Autodesk Inventor part; units mm, degrees
ref_plane "Work Plane1" through (0, 90, 0) normal (1, 0, 0) x (0, 1, 0)
ref_plane "YZ Plane" through (0, 0, 0) normal (1, 0, 0) x (0, 1, 0)
ref_plane "XZ Plane" through (0, 0, 0) normal (0, 1, 0) x (-1, 0, 0)
sketch "Sketch1" plane through (0, 0, 0) normal (1, 0, 0) x (0, 1, 0)
  line L0 (0, 0) -> (90, 0)
  line L1 (90, 0) -> (90, -90)
  line L2 (90, -90) -> (0, -90)
  line L3 (0, -90) -> (0, 0)
  dimension "d0" = 90
  dimension "d1" = 90
ref_plane "Work Plane1" through (0, 90, 0) normal (1, 0, 0) x (0, 1, 0)
sketch "Sketch2" plane through (0, 90, 0) normal (1, 0, 0) x (0, 1, 0)
  line L0 (20, -20) -> (-65, -20)
  line L1 (-65, -20) -> (-65, 0)
  line L2 (-65, 0) -> (-90, 0)
  line L3 (-90, 0) -> (-90, -90)
  line L4 (-90, -90) -> (-65, -90)
  line L5 (-65, -90) -> (-65, -70)
  line L6 (-65, -70) -> (20, -70)
  line L7 (20, -70) -> (20, -20)
  line L8 (0, -90) -> (0, 0)
  line L9 (0, 0) -> (0, -90)
  line L10 (-90, 0) -> (-90, -90)
  line L11 (0, -90) -> (-90, -90)
  line L12 (-90, -90) -> (-90, 0)
  line L13 (-90, 0) -> (0, 0)
  line L14 (0, -45) -> (-90, -45) construction
  circle A0 centre (0, -45) radius 10
  point P0 (20, -45)
  point P1 (-90, -45)
  point P2 (0, -70)
  point P3 (-65, 0)
  point P4 (0, -20)
  point P5 (0, -35)
  point P6 (0, -55)
  dimension "d4" = 90
  dimension "d7" = 50
  dimension "d10" = 20
  dimension "d11" = 90
  dimension "d13" = 25
  dimension "d14" = 25
  dimension "d27" = 110
ref_plane "Work Plane2" through (45, 110, -45) normal (0, 0, 1) x (1, 0, 0)
sketch "Sketch4" plane through (45, 110, -45) normal (0, 0, 1) x (1, 0, 0)
  line L0 (-90, 0) -> (0, 0)
  line L1 (-90, 0) -> (0, 0)
  line L2 (0, 0) -> (0, -110)
  line L3 (0, -110) -> (-90, -110)
  line L4 (-90, -110) -> (-90, 0)
  line L5 (-90, 0) -> (-75, 0)
  line L6 (-75, 0) -> (-15, 0)
  line L7 (-15, 0) -> (0, 0)
  line L8 (0, -110) -> (0, 0)
  line L9 (0, -110) -> (0, -85)
  line L10 (0, -85) -> (-90, -85)
  line L11 (-75, 0) -> (-75, -85)
  line L12 (-15, 0) -> (-15, -85)
  point P0 (-45, -110)
  dimension "d22" = 15
  dimension "d23" = 60
  dimension "d24" = 25
  dimension "d28" = 110
extrude "Extrusion6" add sketch "Sketch2" along normal mid plane 90 contours L7 L6 L8 A0 L0 | L8 A0 L6 L5 L4 L3 L2 L1 L0
extrude "Extrusion7" cut sketch "Sketch4" along normal mid plane 90 contours L0 L12 L10 L11
properties part number "CT_01"
Read the model definition and answer for the solid it produces. Units are mm, in the model's axes. A direction names the side the tool comes from. Round coordinates to 2 decimals unless told otherwise and drop trailing zeros. Loops run counter-clockwise (first coordinate to the right, second up) from the corner with the lowest first, then second, coordinate; pieces in that order, holes last.
Q1. Consider probe 1 along X at (y, z) = (67, -62); probe 2 along Z at (x, y) = (36, 90); probe 3 along Y at (x, z) = (33.75, -45). Determine where each line is inside the solid, lowest interval first.
Q2. Section A-A on y = 62.5 is taken. Write down the section's boundary in (x, z).
Q3. Section D-D on z = -25 is taken. Write down the section's boundary in (x, y), and give its area (3 significant figures).
Q4. Determine the mould class of faces 1 (the face through (-45, 42, -44)), 2 (the face through (-1, 25, -46)), 3 (the face through (37, 68, -20)) for opening direction X: released by +X, released by -X, zero draft, split by the parting line, or undercut.
Q5. Each of these flat-tipped pins is pushed along its axis until it touches: pin 1 (12 mm diameter, centred on x = -40.5, y = 54, fed in from -Z); pin 2 (16.5 mm diameter, centred on x = 38.5, y = 83.5, fed in from +Z); pin 3 (18 mm diameter, centred on y = 90, z = -45, fed in from +X) (1 decimal). Where does it stop, or does it pass through?
Q6. Section B-B on z = -45 is taken. Write down the section's boundary in (x, y), and give its area (3 significant figures).
Q7. Which of the six approach directions +Z, -Z, +X, -X, +Y, -Y give full straight-line access (tool end or side, diameter ignored) to faces 4 (the face through (37, 110, -45)), 5 (the face through (-30, 68, -45)), 6 (the face through (37, 67, -70)), 7 (the face through (-38, 68, -20))?
Q8. Section C-C on y = 90 is taken. Write down the section's boundary in (x, z).
Output:
1. probe 1: x = -45 to -30, 30 to 45
1. probe 2: z = -70 to -55, -35 to -20
1. probe 3: y = 0 to 80, 100 to 110
2. outline: (-45, -70) - (-30, -70) - (-30, -20) - (-45, -20) - close; (30, -70) - (45, -70) - (45, -20) - (30, -20) - close
3. outline: (-45, 0) - (45, 0) - (45, 110) - (30, 110) - (30, 25) - (-30, 25) - (-30, 110) - (-45, 110) - close
3. area: 4,800 mm2
4. face 1: released by -X
4. face 2: undercut
4. face 3: zero draft
5. pin 1: stops at z = -70
5. pin 2: stops at z = -20
5. pin 3: passes through
6. outline: (-45, 0) - (45, 0) - (45, 80) - (30, 80) - (30, 25) - (-30, 25) - (-30, 80) - (-45, 80) - close; (-45, 100) - (-30, 100) - (-30, 110) - (-45, 110) - close; (30, 100) - (45, 100) - (45, 110) - (30, 110) - close
6. area: 4,200 mm2
7. face 4: +Z, -Z, +X, -X, +Y
7. face 5: +Z, -Z, +Y
7. face 6: -Z, +X, -X, +Y
7. face 7: +Z, +X, -X, +Y
8. outline: (-45, -70) - (-30, -70) - (-30, -55) - (-45, -55) - close; (-45, -35) - (-30, -35) - (-30, -20) - (-45, -20) - close; (30, -70) - (45, -70) - (45, -55) - (30, -55) - close; (30, -35) - (45, -35) - (45, -20) - (30, -20) - close
